Can you work these out from the model? Positions are in its coordinate system, mm. A direction names the side the tool comes from. Round coordinates to 2 decimals unless told otherwise and drop trailing zeros. Write each loop counter-clockwise with the first axis right and the second up, starting at its lowest first coordinate (ties: lowest second). Pieces come first, ordered by that corner, then holes.
Q1. If we section it at B-B (y = -73.5): Please give me the cut outline in (x, z), plus the area to 3 significant figures.
Q2. I'm going to push flat-ended pins straight in: pin 1 Ø12 at (y, z) = (-27.5, -181) entering from -X; pin 2 Ø5.5 at (y, z) = (-7.5, 503.5) entering from -X; pin 3 Ø21 at (x, y) = (-39, -10.5) entering from -Z. Where does each tip first touch, or does it pass through?
Q3. Please list where these lines run through material, in increasing order: line 1 along Y through (x, z) = (-187.5, -307); line 2 along X through (y, z) = (-6, 212); line 3 along X through (y, z) = (-18, 200).
Q4. If we section it at A-A (x = 20): Please give me the cut outline in (y, z).
Q5. We'd pull the mould along X, two halves only. Please class faces 6 (the flat face through (-306.83, -9.39, 482.42)), 7 (the flat face through (225, -95.25, 493)), 8 (the cylindrical face through (-238.4, -9.4, 518.8)): +X half, -X half, draft (parallel to the pull), parting line (faces both ways), or undercut.
Q6. For faces 1 (the cylindrical face through (-72.79, -9.39, 518.34)), 2 (the flat face through (282.45, -9.39, 526.78)), 3 (the flat face through (-319.709, -10, 508)), 4 (the flat face through (-73.345, -9.392, 25.362)), 5 (the cylindrical face through (-275.96, -57.68, -432.73)), which set-ups out of +Z, -Z, +X, -X, +Y, -Y let a thin tool reach every point of the face, with its end or its side?
Q7. If we section it at C-C (z = -127): Please give me the cut outline in (x, y), plus the area to 3 significant figures.
from build123d import *

# Parameters (mm, degrees)
F1_DEPTH    = 19.05
F3_DEPTH    = 19.05
F5_D        = 25.8064
F7_R        = 20.5102138496
F7_R_2      = 18.7123578019
F8_DEPTH    = 76.2
F9_T1_DEPTH = 149.6914957887
F9_T3_DEPTH = 96.8143860217
F9_T5_DEPTH = 241.603940201


# Not quite as in the source:
# - a fillet or chamfer that OpenCascade refuses, or shapes differently, is made with other operations: its cross-section is extruded or revolved along the edge and cut away or added


with BuildPart() as f1:
    # F0 (on Front) → F1 (new body)
    with BuildSketch(Plane.XZ):
        Polygon((315.2909820045, 546.1), (227.30280098, 546.1), (-359.2850725167, -469.9), (-271.2968914922, -469.9), align=None)
    extrude(amount=F1_DEPTH)

    # F2 (on face) → F3 (join, through all)
    with BuildSketch(Plane.XZ.offset(19.05)):
        Polygon((227.30280098, 546.1), (-319.7090179955, 546.1), (-319.7090179955, 469.9), (183.3087104677, 469.9), align=None)
    extrude(amount=-F3_DEPTH)

    # F5 (through all)
    with Locations(Plane.XZ.offset(19.05)):
        with Locations((-240.0867491961, 506.0059428215), (-74.4647756219, 505.5469870567), (125.6440877914, 504.5655369759)):
            Hole(F5_D / 2)

    # F7 (on offset) → F8 (join, through all)
    with BuildSketch(Plane.XZ.offset(95.25)):
        with Locations((224.993377924, 492.937207222)):
            Circle(F7_R)
        with Locations((-293.2454049587, -425.5582988262)):
            Circle(F7_R_2)
    extrude(amount=-F8_DEPTH)

    # F9: chamfer of 25.4 on 5 edges, made by hand

    # F9_s2 → F9_t1 (cut)
    with BuildSketch(Plane.XZ.offset(-65.3207478943)):
        Polygon((-294.3090179955, 546.1), (-319.7090179955, 520.7), (-319.7090179955, 546.1), align=None)
        Polygon((-294.3090179955, 469.9), (-319.7090179955, 495.3), (-319.7090179955, 469.9), align=None)
    extrude(amount=F9_T1_DEPTH, mode=Mode.SUBTRACT)

    # F9_s4 → F9_t3 (cut)
    with BuildSketch(Plane.XZ.offset(-38.8821930109)):
        Polygon((-285.9615883296, -469.9), (-263.9645430735, -457.2), (-271.2968914922, -469.9), align=None)
    extrude(amount=F9_T3_DEPTH, mode=Mode.SUBTRACT)

    # F9_s6 → F9_t5 (cut)
    with BuildSketch(Plane.XZ.offset(-111.2769701005)):
        Polygon((293.2939367483, 508), (271.2968914922, 546.1), (315.2909820045, 546.1), align=None)
        Polygon((-315.2909820045, -469.9), (-337.2880272606, -431.8), (-359.2850725167, -469.9), align=None)
    extrude(amount=F9_T5_DEPTH, mode=Mode.SUBTRACT)


solid = f1.part
A:
1. outline: circle Ø37.42 at (-293.25, -425.56); circle Ø41.02 at (224.99, 492.94)
1. area: 2,420 mm2
2. pin 1: passes through
2. pin 2: stops at x = -319.71
2. pin 3: stops at z = -85.74
3. line 1: y = -19.05 to 0
3. line 2: x = 34.41 to 122.4
3. line 3: x = 27.48 to 115.47
4. outline: (-19.05, 34.64) - (0, 34.64) - (0, 187.04) - (-19.05, 187.04) - close; (-19.05, 469.9) - (0, 469.9) - (0, 546.1) - (-19.05, 546.1) - close
5. face 6: -X half
5. face 7: draft
5. face 8: undercut
6. face 1: +Y, -Y
6. face 2: +Z, +X, +Y, -Y
6. face 3: +Z, -X, +Y, -Y
6. face 4: -X, +Y, -Y
6. face 5: -Y
7. outline: (-161.31, -19.05) - (-73.32, -19.05) - (-73.32, 0) - (-161.31, 0) - close
7. area: 1,680 mm2
